Autodesk Inventor part; units mm, degrees
ref_plane "YZ Plane" through (0, 0, 0) normal (1, 0, 0) x (0, 1, 0)
ref_plane "XZ Plane" through (0, 0, 0) normal (0, 1, 0) x (-1, 0, 0)
ref_plane "XY Plane" through (0, 0, 0) normal (0, 0, 1) x (1, 0, 0)
sketch "Sketch1" plane through (0, 0, 0) normal (0, 0, 1) x (1, 0, 0)
  line L0 (0, 0) -> (6.1915, 5.0087)
  line L1 (6.1915, 5.0087) -> (12.383, 0)
  line L2 (12.383, 0) -> (0, -13.1985)
  line L3 (0, -13.1985) -> (0, 0)
  point P0 (5.6638, -7.1617)
  dimension "d2" = 7.854
  dimension "d3" = 7.9638
  dimension "d4" = 18.0981
extrude "Extrusion1" add sketch "Sketch1" along normal blind 10
sketch "Sketch3" plane through (0, 0, 10) normal (-0.6289, 0.7775, 0) x (0, 0, -1)
  circle A0 centre (4.9487, 0) radius 3.2373
  point P0 (10, 0)
extrude "Extrusion2" cut sketch "Sketch3" against normal blind 10
fillet "Fillet1" radius 2.02 2 edges at (9.2873, 2.5044, 10) (9.2873, 2.5044, 0)
properties part number "My really cool, really epic hole in a ramp"
Can you work these out from the model? Positions are in its coordinate system, mm. Round coordinates to 2 decimals unless told otherwise and drop trailing zeros. Write each loop counter-clockwise with the first axis right and the second up, starting at its lowest first coordinate (ties: lowest second). Pieces come first, ordered by that corner, then holes. Notation, with made-up numbers: (-39, -17) - (11, -17) arc R27 ccw to (11, 18) - close; hole circle Ø1 at (70.5, 56.5). An arc over 180 degrees is marked (long way). Write each question's results on one line, items separated by ' | '. Start each with the question number.
1) Suppose I cut it at A-A (z = 4.25). List the corners of the cut face in (x, y) for me, and give its area (3 significant figures).
2) We'd pull the mould along Y, two halves only. Please class faces 1 (the cylindrical face through (5.422, -1.679, 5.753)), 2 (the flat face through (7.654, -5.04, 2.708)), 3 (the flat face through (4, -3, 0)): released by +Y, released by -Y, zero draft, split by the parting line, or undercut.
3) For pin 1 Ø1 at (x, z) = (7.5, 9) entering from +Y; pin 2 Ø5 at (y, z) = (-11, 6) entering from +X; pin 3 Ø3 at (y, z) = (-3, 3.5) entering from +X, each with a flat end and sliding along its axis, tell me the tip position at first contact or that it passes through.
4) Suppose I cut it at B-B (z = 5.5). List the corners of the cut face in (x, y) for me, and give its area (3 significant figures).
5) Please list where these lines run through material, in increasing order: line 1 (Y direction, x = 1.5, z = 7.75); line 2 (Y direction, x = 3.25, z = 4); line 3 (Z direction, x = 1.5, y = -0.25).
6) Suppose I cut it at C-C (z = 0.5). List the corners of the cut face in (x, y) for me, and give its area (3 significant figures).
Here are the results:
1) outline: (0, -13.2) - (3.57, -9.4) - (0, -4.99) - close; (2.44, 1.97) - (7.9, -4.78) - (12.38, 0) - (6.19, 5.01) - close | area: 61.6 mm2
2) face 1: undercut | face 2: released by -Y | face 3: zero draft
3) pin 1: stops at y = 4.1 | pin 2: stops at x = 4.09 | pin 3: stops at x = 10.98
4) outline: (0, -13.2) - (3.52, -9.45) - (0, -5.1) - close; (2.49, 2.02) - (7.95, -4.73) - (12.38, 0) - (6.19, 5.01) - close | area: 60.6 mm2
5) line 1: y = -11.6 to -4.7, 0.99 to 1.21 | line 2: y = -9.73 to -8.89, 0.85 to 2.63 | line 3: z = 0 to 1.98, 8.13 to 10
6) outline: (0, -13.2) - (11.91, -0.5) - (5.64, 4.57) - (0, 0) - close | area: 107 mm2
